Model file for the job. Use its own axes, mm. A direction names the side the tool comes from. Coordinates: 2 decimals unless noted, no trailing zeros. Write each loop counter-clockwise with the first axis right and the second up, starting at its lowest first coordinate (ties: lowest second). Pieces come first, ordered by that corner, then holes. Notation, with made-up numbers: (-6, 61.5) -> (20, 61.5) arc R16 cw to (20, 81.5) -> close; hole circle Ø10 at (45, 70). An arc over 180 degrees is marked (long way). Answer as a JSON object with one key per item and string values. Group by question number.
from build123d import *

# Parameters (mm, degrees)
F1_DEPTH  = 3.25
F3_DEPTH  = 1
F5_DEPTH  = 1
F7_DEPTH  = 0.5
F9_DEPTH  = 0.5
F10_W     = 24
F10_H     = 2.8
F11_DEPTH = 20
F13_DEPTH = 1.4
F14_W     = 8
F14_H     = 1
F15_DEPTH = 25
F16_R     = 1


with BuildPart() as f1:
    # F0 (on Front) → F1 (new body, symmetric)
    with BuildSketch(Plane.XZ):
        Polygon((18, 18), (0, 18), (-18, 18), (-35, 0), (0, -47), (35, 0), align=None)
    extrude(amount=F1_DEPTH, both=True)

    # F2 (on face) → F3 (cut)
    with BuildSketch(Plane.XZ.offset(3.25)):
        Polygon((15.844768, 13), (-15.844768, 13), (-28.482277, -0.380893), (0, -38.628523), (28.482278, -0.380893), align=None)
    extrude(amount=-F3_DEPTH, mode=Mode.SUBTRACT)

    # F4 (on face) → F5 (cut)
    with BuildSketch(Plane(origin=(0, 3.25, 0), x_dir=(-1, 0, 0), z_dir=(0, 1, 0))):
        Polygon((28.482278, -0.380893), (15.844768, 13), (-15.844767, 13), (-28.482277, -0.380893), (0, -38.628522), align=None)
    extrude(amount=-F5_DEPTH, mode=Mode.SUBTRACT)

    # F6 (on face) → F7 (join)
    with BuildSketch(Plane(origin=(0, 2.25, 0), x_dir=(-1, 0, 0), z_dir=(0, 1, 0))):
        with BuildLine():
            Line((15.844768, 13), (11.844768, 13))
            Line((11.844768, 13), (11.844768, 12.5))
            Line((11.844768, 12.5), (-11.844768, 12.5))
            Line((-11.844768, 12.5), (-11.844768, 13))
            Line((-11.844768, 13), (-15.844768, 13))
            Line((-15.844768, 13), (-15.844768, 8))
            Line((-15.844768, 8), (-11.844768, 8))
            Line((-11.844768, 8), (-11.844768, 8.5))
            Line((-11.844768, 8.5), (11.844768, 8.5))
            Line((11.844768, 8.5), (11.844768, -11))
            ThreePointArc((11.844768, -11), (0, -22.844768), (-11.844768, -11))
            Line((-11.844768, -11), (-15.844768, -11))
            ThreePointArc((-15.844768, -11), (0, -26.844768), (15.844768, -11))
            Line((15.844768, -11), (15.844768, 13))
        make_face()
    extrude(amount=F7_DEPTH)

    # F8 (on face) → F9 (join)
    with BuildSketch(Plane.XZ.offset(2.25)):
        with BuildLine():
            Line((15.844768, 13), (11.844768, 13))
            Line((11.844768, 13), (11.844768, 12.500001))
            Line((11.844768, 12.500001), (-11.844767, 12.500001))
            Line((-11.844767, 12.500001), (-11.844767, 13))
            Line((-11.844767, 13), (-15.844767, 13))
            Line((-15.844767, 13), (-15.844767, 8.000001))
            Line((-15.844767, 8.000001), (-11.844767, 8.000001))
            Line((-11.844767, 8.000001), (-11.844767, 8.500001))
            Line((-11.844767, 8.500001), (11.844768, 8.500001))
            Line((11.844768, 8.500001), (11.844768, -11))
            ThreePointArc((11.844768, -11), (0, -22.844767), (-11.844767, -11))
            Line((-11.844767, -11), (-15.844767, -11))
            ThreePointArc((-15.844767, -11), (0, -26.844767), (15.844768, -11))
            Line((15.844768, -11), (15.844768, 13))
        make_face()
    extrude(amount=F9_DEPTH)

    # F10 (on face) → F11 (cut)
    with BuildSketch(Plane.XY.offset(18)):
        Rectangle(F10_W, F10_H)
    extrude(amount=-F11_DEPTH, mode=Mode.SUBTRACT)

    # F12 (on Front) → F13 (cut, symmetric)
    with BuildSketch(Plane.XZ):
        with BuildLine():
            Line((12, -2), (-12, -2))
            ThreePointArc((-12, -2), (0, -14), (12, -2))
        make_face()
    extrude(amount=F13_DEPTH, both=True, mode=Mode.SUBTRACT)

    # F14 (on face) → F15 (cut)
    with BuildSketch(Plane.XZ.offset(3.25)):
        with Locations((0, 15.5)):
            Rectangle(F14_W, F14_H)
    extrude(amount=-F15_DEPTH, mode=Mode.SUBTRACT)

    # F16
    f16_edges = [f1.edges().sort_by_distance(p)[0] for p in [
        (0, 0, -47),
        (35, 0, 0),
        (-35, 0, 0),
        (-18, 0, 18),
        (18, 0, 18),
    ]]
    fillet(f16_edges, radius=F16_R)


solid = f1.part
(1) Cut at A-A on y = 0. List the corners of the cut face in (x, z).
(2) Pin check, flat tips, straight feed: pin 1 (3 mm diameter, centred on y = -1.5, z = -36.5, fed in from +X); pin 2 (2 mm diameter, centred on x = 18, z = -9, fed in from +Y); pin 3 (2 mm diameter, centred on y = 0, z = 3.5, fed in from -X). Stop position of each tip, or through.
(3) Pull direction Z, two halves, no side cores. Call faces 1 (the face through (0, 2, 16)), 2 (the face through (26.5, 0, 9)), 3 (the face through (12, 0, 8)): released by +Z, released by -Z, zero draft, split by the parting line, or undercut.
(4) Cut at B-B on z = -7.5. List the corners of the cut face in (x, y).
(5) 3-axis set-ups, long thin cutter, end or side, ignore diameter. For faces 4 (the face through (22.25, -2.76, 6.22)), 5 (the face through (-26.247, -0.046, 9.268)), 6 (the face through (0, 1.4, 2)), 7 (the face through (14.44, 2.76, -19.24)), 8 (the face through (0, 2, 15)): which of +Z, -Z, +X, -X, +Y, -Y reach the whole face in a straight line?
(6) Wall check: probe 1 along Y at (x, z) = (3.5, -8); probe 2 along X at (y, z) = (-2.5, 5.5); probe 3 along X at (y, z) = (-2.5, -19). Give the ranges that are in metal, low to high.
(7) Cut at C-C on x = 24. List the corners of the cut face in (y, z), plus the area to 3 significant figures.
(8) Cut at D-D on z = -37. List the corners of the cut face in (x, y), plus the area to 3 significant figures.
Results found:
{
 "1": {"outline": "(-34.5, -0.67) -> (-0.8, -45.92) arc R1 ccw to (0.8, -45.92) -> (34.5, -0.67) arc R1 ccw to (34.42, 0.61) -> (18.3, 17.69) arc R1 ccw to (17.57, 18) -> (12, 18) -> (12, -2) arc R12 cw to (-12, -2) -> (-12, 18) -> (-17.57, 18) arc R1 ccw to (-18.3, 17.69) -> (-34.42, 0.61) arc R1 ccw to start"},
 "2": {"pin 1": "stops at x = 8.94", "pin 2": "stops at y = 2.25", "pin 3": "stops at x = -32.64"},
 "3": {"face 1": "undercut", "face 2": "released by +Z", "face 3": "zero draft"},
 "4": {"outline": "(-29.41, -3.25) -> (-23.18, -3.25) -> (-23.18, -2.25) -> (11.84, -2.25) -> (11.84, -2.75) -> (15.84, -2.75) -> (15.84, -2.25) -> (23.18, -2.25) -> (23.18, -3.25) -> (29.41, -3.25) -> (29.41, 3.25) -> (23.18, 3.25) -> (23.18, 2.25) -> (-11.84, 2.25) -> (-11.84, 2.75) -> (-15.84, 2.75) -> (-15.84, 2.25) -> (-23.18, 2.25) -> (-23.18, 3.25) -> (-29.41, 3.25) -> close; hole (-10.67, -1.4) -> (10.67, -1.4) -> (10.67, 1.4) -> (-10.67, 1.4) -> close"},
 "5": {"face 4": "-Y", "face 5": "+Z, -X, +Y, -Y", "face 6": "+Z", "face 7": "+Y", "face 8": "+Y, -Y"},
 "6": {"probe 1": "y = -2.25 to -1.4, 1.4 to 2.25", "probe 2": "x = -29.81 to -22.93, 11.84 to 15.84, 22.93 to 29.81", "probe 3": "x = -20.85 to -14.62, -13.68 to -8.73, 8.73 to 13.68, 14.62 to 20.85"},
 "7": {"outline": "(-3.25, -14.77) -> (3.25, -14.77) -> (3.25, -6.4) -> (2.25, -6.4) -> (2.25, 4.37) -> (3.25, 4.37) -> (3.25, 11.65) -> (-3.25, 11.65) -> (-3.25, 4.37) -> (-2.25, 4.37) -> (-2.25, -6.4) -> (-3.25, -6.4) -> close", "area": "150 mm²"},
 "8": {"outline": "(-7.45, -3.25) -> (-1.21, -3.25) -> (-1.21, -2.25) -> (1.21, -2.25) -> (1.21, -3.25) -> (7.45, -3.25) -> (7.45, 3.25) -> (1.21, 3.25) -> (1.21, 2.25) -> (-1.21, 2.25) -> (-1.21, 3.25) -> (-7.45, 3.25) -> close", "area": "92.0 mm²"}
}
